The listing builds one solid part. Answer for the finished solid, in the listing's coordinates (mm). A direction names the side the tool comes from. Give positions to 0.01 mm unless a question says otherwise; leave off trailing zeros. Write each loop counter-clockwise with the first axis right and the second up, starting at its lowest first coordinate (ties: lowest second). Pieces come first, ordered by that corner, then holes. Notation, with made-up numbers: (15.25, 55.5) - (37.25, 55.5) arc R6 cw to (37.25, 64.5) - close; hole circle Ø11 at (-15.75, -19.5). An arc over 180 degrees is marked (long way). Use a Markdown table: item, result. Add a question column.
from build123d import *

# Parameters (mm, degrees)
F0_W      = 23
F0_H      = 25
F1_DEPTH  = 7
F3_DEPTH  = 25.001
F4_DEPTH  = 12.5
F5_SIZE   = 6
F6_R      = 10
F7_R      = 1.6
F8_DEPTH  = 25
F10_DEPTH = 2.5


with BuildPart() as f1:
    # F0 (on Top) → F1 (new body)
    with BuildSketch(Plane.XY):
        Rectangle(F0_W, F0_H)
    extrude(amount=F1_DEPTH)

    # F2 (on face) → F3 (cut, through all)
    with BuildSketch(Plane.XZ.offset(12.5)):
        with BuildLine():
            Line((0, 7), (-2.2912878475, 7))
            ThreePointArc((-2.2912878475, 7), (0, 5.5), (2.2912878475, 7))
            Line((2.2912878475, 7), (0, 7))
        make_face()
    extrude(amount=-F3_DEPTH, mode=Mode.SUBTRACT)

    # F2 (on face) → F4 (cut)
    with BuildSketch(Plane.XZ.offset(12.5)):
        with BuildLine():
            ThreePointArc((2.2912878475, 7), (0, 5.5), (-2.2912878475, 7))
            Line((-2.2912878475, 7), (-2.8084005449, 7))
            Line((-2.8084005449, 7), (-3.0722061624, 6.9397880893))
            ThreePointArc((-3.0722061624, 6.9397880893), (-2.9281488207, 6.5898778479), (-2.7443962613, 6.2590838157))
            Line((-2.7443962613, 6.2590838157), (-2.4464411557, 6.4966950836))
            Line((-2.4464411557, 6.4966950836), (-2.0099982944, 5.9494130458))
            Line((-2.0099982944, 5.9494130458), (-2.3079534, 5.711801778))
            ThreePointArc((-2.3079534, 5.711801778), (-2.026341856, 5.459047682), (-1.7172603691, 5.2407398048))
            Line((-1.7172603691, 5.2407398048), (-1.5519077603, 5.5840980352))
            Line((-1.5519077603, 5.5840980352), (-0.9212295527, 5.2803794178))
            Line((-0.9212295527, 5.2803794178), (-1.0865821616, 4.9370211875))
            ThreePointArc((-1.0865821616, 4.9370211875), (-0.7231930354, 4.8314842854), (-0.35, 4.7689011157))
            Line((-0.35, 4.7689011157), (-0.35, 5.15))
            Line((-0.35, 5.15), (0.35, 5.15))
            Line((0.35, 5.15), (0.35, 4.7689011157))
            ThreePointArc((0.35, 4.7689011157), (0.7231930354, 4.8314842854), (1.0865821616, 4.9370211875))
            Line((1.0865821616, 4.9370211875), (0.9212295527, 5.2803794178))
            Line((0.9212295527, 5.2803794178), (1.5519077603, 5.5840980352))
            Line((1.5519077603, 5.5840980352), (1.7172603691, 5.2407398048))
            ThreePointArc((1.7172603691, 5.2407398048), (2.026341856, 5.459047682), (2.3079534, 5.711801778))
            Line((2.3079534, 5.711801778), (2.0099982944, 5.9494130458))
            Line((2.0099982944, 5.9494130458), (2.4464411557, 6.4966950836))
            Line((2.4464411557, 6.4966950836), (2.7443962613, 6.2590838157))
            ThreePointArc((2.7443962613, 6.2590838157), (2.9281488207, 6.5898778479), (3.0722061624, 6.9397880893))
            Line((3.0722061624, 6.9397880893), (2.8084005449, 7))
            Line((2.8084005449, 7), (2.2912878475, 7))
        make_face()
        with BuildLine():
            Line((3.0719063417, 5.9979032421), (2.7443962613, 6.2590838157))
            ThreePointArc((2.7443962613, 6.2590838157), (2.540952318, 5.973658144), (2.3079534, 5.711801778))
            Line((2.3079534, 5.711801778), (2.6354634804, 5.4506212044))
            Line((2.6354634804, 5.4506212044), (3.0719063417, 5.9979032421))
        make_face()
        with BuildLine():
            ThreePointArc((2.3079534, 5.711801778), (2.540952318, 5.973658144), (2.7443962613, 6.2590838157))
            Line((2.7443962613, 6.2590838157), (2.4464411557, 6.4966950836))
            Line((2.4464411557, 6.4966950836), (2.0099982944, 5.9494130458))
            Line((2.0099982944, 5.9494130458), (2.3079534, 5.711801778))
        make_face()
        with BuildLine():
            Line((1.8990147515, 4.8633229408), (1.7172603691, 5.2407398048))
            ThreePointArc((1.7172603691, 5.2407398048), (1.4101221521, 5.0718511793), (1.0865821616, 4.9370211875))
            Line((1.0865821616, 4.9370211875), (1.268336544, 4.5596043235))
            Line((1.268336544, 4.5596043235), (1.8990147515, 4.8633229408))
        make_face()
        with BuildLine():
            ThreePointArc((1.0865821616, 4.9370211875), (1.4101221521, 5.0718511793), (1.7172603691, 5.2407398048))
            Line((1.7172603691, 5.2407398048), (1.5519077603, 5.5840980352))
            Line((1.5519077603, 5.5840980352), (0.9212295527, 5.2803794178))
            Line((0.9212295527, 5.2803794178), (1.0865821616, 4.9370211875))
        make_face()
        with BuildLine():
            ThreePointArc((0.35, 4.7689011157), (0, 4.75), (-0.35, 4.7689011157))
            Line((-0.35, 4.7689011157), (-0.35, 4.35))
            Line((-0.35, 4.35), (0.35, 4.35))
            Line((0.35, 4.35), (0.35, 4.7689011157))
        make_face()
        with BuildLine():
            Line((-0.35, 5.15), (-0.35, 4.7689011157))
            ThreePointArc((-0.35, 4.7689011157), (0, 4.75), (0.35, 4.7689011157))
            Line((0.35, 4.7689011157), (0.35, 5.15))
            Line((0.35, 5.15), (-0.35, 5.15))
        make_face()
        with BuildLine():
            ThreePointArc((-1.0865821616, 4.9370211875), (-1.4101221521, 5.0718511793), (-1.7172603691, 5.2407398048))
            Line((-1.7172603691, 5.2407398048), (-1.8990147515, 4.8633229408))
            Line((-1.8990147515, 4.8633229408), (-1.268336544, 4.5596043235))
            Line((-1.268336544, 4.5596043235), (-1.0865821616, 4.9370211875))
        make_face()
        with BuildLine():
            Line((-1.5519077603, 5.5840980352), (-1.7172603691, 5.2407398048))
            ThreePointArc((-1.7172603691, 5.2407398048), (-1.4101221521, 5.0718511793), (-1.0865821616, 4.9370211875))
            Line((-1.0865821616, 4.9370211875), (-0.9212295527, 5.2803794178))
            Line((-0.9212295527, 5.2803794178), (-1.5519077603, 5.5840980352))
        make_face()
        with BuildLine():
            ThreePointArc((-2.3079534, 5.711801778), (-2.540952318, 5.973658144), (-2.7443962613, 6.2590838157))
            Line((-2.7443962613, 6.2590838157), (-3.0719063417, 5.9979032421))
            Line((-3.0719063417, 5.9979032421), (-2.6354634804, 5.4506212044))
            Line((-2.6354634804, 5.4506212044), (-2.3079534, 5.711801778))
        make_face()
        with BuildLine():
            Line((-2.4464411557, 6.4966950836), (-2.7443962613, 6.2590838157))
            ThreePointArc((-2.7443962613, 6.2590838157), (-2.540952318, 5.973658144), (-2.3079534, 5.711801778))
            Line((-2.3079534, 5.711801778), (-2.0099982944, 5.9494130458))
            Line((-2.0099982944, 5.9494130458), (-2.4464411557, 6.4966950836))
        make_face()
        with BuildLine():
            Line((3.0923292192, 7), (2.8084005449, 7))
            Line((2.8084005449, 7), (3.0722061624, 6.9397880893))
            ThreePointArc((3.0722061624, 6.9397880893), (3.0824147168, 6.969844908), (3.0923292192, 7))
        make_face()
        with BuildLine():
            Line((-3.0722061624, 6.9397880893), (-2.8084005449, 7))
            Line((-2.8084005449, 7), (-3.0923292192, 7))
            ThreePointArc((-3.0923292192, 7), (-3.0824147168, 6.969844908), (-3.0722061624, 6.9397880893))
        make_face()
    extrude(amount=-F4_DEPTH, mode=Mode.SUBTRACT)

    # F5
    f5_edges = [f1.edges().sort_by_distance(p)[0] for p in [
        (11.5, -12.5, 3.5),
        (-11.5, -12.5, 3.5),
        (11.5, 12.5, 3.5),
        (-11.5, 12.5, 3.5),
    ]]
    chamfer(f5_edges, length=F5_SIZE)

    # F6
    f6_edges = [f1.edges().sort_by_distance(p)[0] for p in [
        (11.5, 6.5, 3.5),
        (11.5, -6.5, 3.5),
        (-11.5, 6.5, 3.5),
        (-11.5, -6.5, 3.5),
    ]]
    fillet(f6_edges, radius=F6_R)

    # F7 (on face) → F8 (cut)
    with BuildSketch(Plane.XY.offset(7)):
        with Locations((6, -7)):
            Circle(F7_R)
        with Locations((-6, -7)):
            Circle(F7_R)
        with Locations((-6, 7)):
            Circle(F7_R)
        with Locations((6, 7)):
            Circle(F7_R)
    extrude(amount=-F8_DEPTH, mode=Mode.SUBTRACT)

    # F9 (on face) → F10 (cut)
    with BuildSketch(Plane(origin=(0, 0, 0), x_dir=(1, 0, 0), z_dir=(0, 0, -1))):
        Polygon((-4.3545517328, 4.15), (-2.7091034656, 7), (-4.3545517328, 9.85), (-7.6454482672, 9.85), (-9.2908965344, 7), (-7.6454482672, 4.15), align=None)
        Polygon((-9.2908965344, -7), (-7.6454482672, -9.85), (-4.3545517328, -9.85), (-2.7091034656, -7), (-4.3545517328, -4.15), (-7.6454482672, -4.15), align=None)
        Polygon((2.7091034656, 7), (4.3545517328, 4.15), (7.6454482672, 4.15), (9.2908965344, 7), (7.6454482672, 9.85), (4.3545517328, 9.85), align=None)
        Polygon((2.7091034656, -7), (4.3545517328, -9.85), (7.6454482672, -9.85), (9.2908965344, -7), (7.6454482672, -4.15), (4.3545517328, -4.15), align=None)
    extrude(amount=-F10_DEPTH, mode=Mode.SUBTRACT)


solid = f1.part
1. The part is cut by section D-D (y = 7.75). Give the vertices of the cut face in (x, z), and give its area (3 significant figures).
2. Which of the six approach directions +Z, -Z, +X, -X, +Y, -Y give full straight-line access (tool end or side, diameter ignored) to faces 1 (the cylindrical face through (-10.76, -6.13, 3.55)), 2 (the flat face through (6, -9.85, 1))?
3. The part is cut by section C-C (z = 3.25). Give the vertices of the cut face in (x, y).
4. For a pull along X with two mould halves and no side action, classify faces 3 (the cylindrical face through (10.718, 6.235, 3.549)), 4 (the flat face through (-7, 11, 3)), 5 (the flat face through (0, 0, 0)), 6 (the cylindrical face through (-6.35, 5.44, 4.78)) as released by +X, released by -X, zero draft, split by the parting line, or undercut.
5. The part is cut by section A-A (x = 6). Give the vertices of the cut face in (y, z), and give its area (3 significant figures).
6. Given P1, Ø2, axis at x = -2, y = -9.5, coming from the +Z side; P2, Ø1.2, axis at x = 6.5, z = 2, coming from the +Y side; P3, Ø3, axis at x = 6, y = 7, coming from the +Z side; P4, Ø0.5, axis at y = -9.5, z = 4.5, coming from the -X side, each flat-ended and moving along its own axis, determine where each tip first touches the part or whether it passes through.
7. The part is cut by section B-B (y = -10.25). Give the vertices of the cut face in (x, z), and give its area (3 significant figures).
8. Consider L1, parallel to Y at x = 6, z = 5.4; L2, parallel to Y at x = 8, z = 2; L3, parallel to Z at x = -6.75, y = 8.75. Determine where each line is inside the solid, lowest interval first. Write a range as [from, to].
Check values:
| question | item | result |
|---|---|---|
| 1 | outline | (-9.92, 0) - (-8.86, 0) - (-8.86, 2.5) - (-7.41, 2.5) - (-7.41, 7) - (-9.92, 7) - close; (-4.59, 2.5) - (-3.14, 2.5) - (-3.14, 0) - (3.14, 0) - (3.14, 2.5) - (4.59, 2.5) - (4.59, 7) - (2.29, 7) arc R2.5 cw to (-2.29, 7) - (-4.59, 7) - close; (7.41, 2.5) - (8.86, 2.5) - (8.86, 0) - (9.92, 0) - (9.92, 7) - (7.41, 7) - close |
| 1 | area | 79.9 mm2 |
| 2 | face 1 | +Z, -Z, -X, -Y |
| 2 | face 2 | -Z |
| 3 | outline | (-11.5, -2.36) arc R10 ccw to (-8.57, -9.43) - (-5.5, -12.5) - (5.5, -12.5) - (8.57, -9.43) arc R10 ccw to (11.5, -2.36) - (11.5, 2.36) arc R10 ccw to (8.57, 9.43) - (5.5, 12.5) - (-5.5, 12.5) - (-8.57, 9.43) arc R10 ccw to (-11.5, 2.36) - close; hole circle Ø3.2 at (-6, -7); hole circle Ø3.2 at (-6, 7); hole circle Ø3.2 at (6, -7); hole circle Ø3.2 at (6, 7) |
| 4 | face 3 | released by +X |
| 4 | face 4 | released by -X |
| 4 | face 5 | zero draft |
| 4 | face 6 | undercut |
| 5 | outline | (-12, 0) - (-9.85, 0) - (-9.85, 2.5) - (-8.6, 2.5) - (-8.6, 7) - (-12, 7) - close; (-5.4, 2.5) - (-4.15, 2.5) - (-4.15, 0) - (4.15, 0) - (4.15, 2.5) - (5.4, 2.5) - (5.4, 7) - (-5.4, 7) - close; (8.6, 2.5) - (9.85, 2.5) - (9.85, 0) - (12, 0) - (12, 7) - (8.6, 7) - close |
| 5 | area | 111 mm2 |
| 6 | P1 | stops at z = 6.75 |
| 6 | P2 | stops at y = 12.1 |
| 6 | P3 | passes through |
| 6 | P4 | stops at x = -8.75 |
| 7 | outline | (-7.75, 0) - (7.75, 0) - (7.75, 7) - (3.09, 7) arc R3.25 cw to (2.74, 6.26) - (3.07, 6) - (2.64, 5.45) - (2.31, 5.71) arc R3.25 cw to (1.72, 5.24) - (1.9, 4.86) - (1.27, 4.56) - (1.09, 4.94) arc R3.25 cw to (0.35, 4.77) - (0.35, 4.35) - (-0.35, 4.35) - (-0.35, 4.77) arc R3.25 cw to (-1.09, 4.94) - (-1.27, 4.56) - (-1.9, 4.86) - (-1.72, 5.24) arc R3.25 cw to (-2.31, 5.71) - (-2.64, 5.45) - (-3.07, 6) - (-2.74, 6.26) arc R3.25 cw to (-3.09, 7) - (-7.75, 7) - close |
| 7 | area | 96.9 mm2 |
| 8 | L1 | y = [-12, -8.6], [-5.4, 5.4], [8.6, 12] |
| 8 | L2 | y = [-10, -9.24], [-4.76, 4.76], [9.24, 10] |
| 8 | L3 | z = [2.5, 7] |
